```python
from build123d import *

# Parameters (mm, degrees)
F0_R     = 14.2875
F1_DEPTH = 28.448
F0_R_2   = 6.35
F2_DEPTH = 11.176
F3_R     = 3.302


with BuildPart() as f1:
    # F0 (on Top) → F1 (new body)
    with BuildSketch(Plane.XY):
        with BuildLine():
            ThreePointArc((25.4, 61.976), (0, 87.376), (-25.4, 61.976))
            ThreePointArc((-25.4, 61.976), (0, 36.576), (25.4, 61.976))
        make_face()
        with Locations((0, 61.976)):
            Circle(F0_R, mode=Mode.SUBTRACT)
    extrude(amount=F1_DEPTH)

    # F0 (on Top) → F2 (join)
    with BuildSketch(Plane.XY):
        with BuildLine():
            Line((-28.575, 0), (0, 0))
            Line((0, 0), (28.575, 0))
            ThreePointArc((28.575, 0), (45.1140748574, 9.5968786709), (44.989265753, 28.7182149226))
            Line((44.989265753, 28.7182149226), (25.4, 61.976))
            ThreePointArc((25.4, 61.976), (0, 36.576), (-25.4, 61.976))
            Line((-25.4, 61.976), (-44.989265753, 28.7182149226))
            ThreePointArc((-44.989265753, 28.7182149226), (-45.1140748574, 9.5968786709), (-28.575, 0))
        make_face()
        with Locations((-28.575, 19.05)):
            Circle(F0_R_2, mode=Mode.SUBTRACT)
        with Locations((28.575, 19.05)):
            Circle(F0_R_2, mode=Mode.SUBTRACT)
    extrude(amount=F2_DEPTH)

    # F3
    f3_edges = [f1.edges().sort_by_distance(p)[0] for p in [
        (25.4, 61.976, 28.448),
    ]]
    fillet(f3_edges, radius=F3_R)


solid = f1.part
```
Build history of the part. All positions in model axes, mm. A direction names the side the tool comes from. Round coordinates to 2 decimals unless told otherwise and drop trailing zeros. Write each loop counter-clockwise with the first axis right and the second up, starting at its lowest first coordinate (ties: lowest second). Pieces come first, ordered by that corner, then holes. Notation, with made-up numbers: (-31, 86) - (23, 86) arc R29 cw to (23, 115) - close; hole circle Ø8 at (-5.75, 47.5). An arc over 180 degrees is marked (long way). Write each question's results on one line, items separated by ' | '. Start each with the question number.
Item 1: Saw through at D-D (z = 20.75). Write the cut outline in (x, y) (1 decimal).
Item 2: Which spindle directions (+Z, -Z, +X, -X, +Y, -Y) get a long thin tool onto all of the face, cutting with end or side? Do faces 5 (the face through (-22.52, 20.96, 5.51)), 6 (the face through (5.51, 86.77, 15.19)). Say none if no direction does.
Item 3: Wall check: L1, parallel to X at y = 23, z = 3.5; L2, parallel to Z at x = -36.5, y = 36.5; L3, parallel to X at y = 63, z = 8. Give the ranges that are in metal, low to high. Write a range as [from, to].
Item 4: Mould opens along X. For faces 1 (the face through (5, 48, 28.448)), 2 (the face through (-3.1, 48.03, 14.02)), 3 (the face through (35.332, 45.114, 5.51)), 4 (the face through (-35.058, 45.58, 5.51)) say: pulls with the +X half, pulls with the -X half, needs draft (parallel to the pull), parting line crosses it, or undercut.
Item 5: Saw through at B-B (z = 9.5). State how many separate pieces and enclosed holes the cut face has, and give its area (3 significant figures).
Item 6: Saw through at A-A (x = 0). Write the cut outline in (y, z), and give its area (3 significant figures).
Item 7: Saw through at C-C (y = 19.05). Write the cut outline in (x, z) (3 decimals), and give its area (3 significant figures).
Item 8: Drop flat-ended pins along their axis: P1, Ø3, axis at y = 15.5, z = 3.5, coming from the -X side; P2, Ø5, axis at x = 38, y = 40, coming from the +Z side; P3, Ø3, axis at x = 16.5, y = 55.5, coming from the -Z side; P4, Ø8, axis at y = 70.5, z = 10.5, coming from the +X side. Give the stop position or say it passes through.
Results are:
1) outline: circle Ø50.8 at (0, 62); hole circle Ø28.6 at (0, 62)
2) face 5: +Z, -Z | face 6: +Z
3) L1: x = [-47.21, -33.55], [-23.6, 23.6], [33.55, 47.21] | L2: z = [0, 11.18] | L3: x = [-25.38, -14.25], [14.25, 25.38]
4) face 1: needs draft | face 2: undercut | face 3: pulls with the +X half | face 4: pulls with the -X half
5) separate pieces: 1 | enclosed holes: 3 | area: 5,020 mm²
6) outline: (0, 0) - (47.69, 0) - (47.69, 28.45) - (39.88, 28.45) arc R3.3 ccw to (36.58, 25.15) - (36.58, 11.18) - (0, 11.18) - close; (76.26, 0) - (87.38, 0) - (87.38, 25.15) arc R3.3 ccw to (84.07, 28.45) - (76.26, 28.45) - close | area: 1,040 mm²
7) outline: (-47.625, 0) - (-34.925, 0) - (-34.925, 11.176) - (-47.625, 11.176) - close; (-22.225, 0) - (22.225, 0) - (22.225, 11.176) - (-22.225, 11.176) - close; (34.925, 0) - (47.625, 0) - (47.625, 11.176) - (34.925, 11.176) - close | area: 781 mm²
8) P1: stops at x = -47.51 | P2: stops at z = 11.18 | P3: stops at z = 0 | P4: stops at x = 24.99
